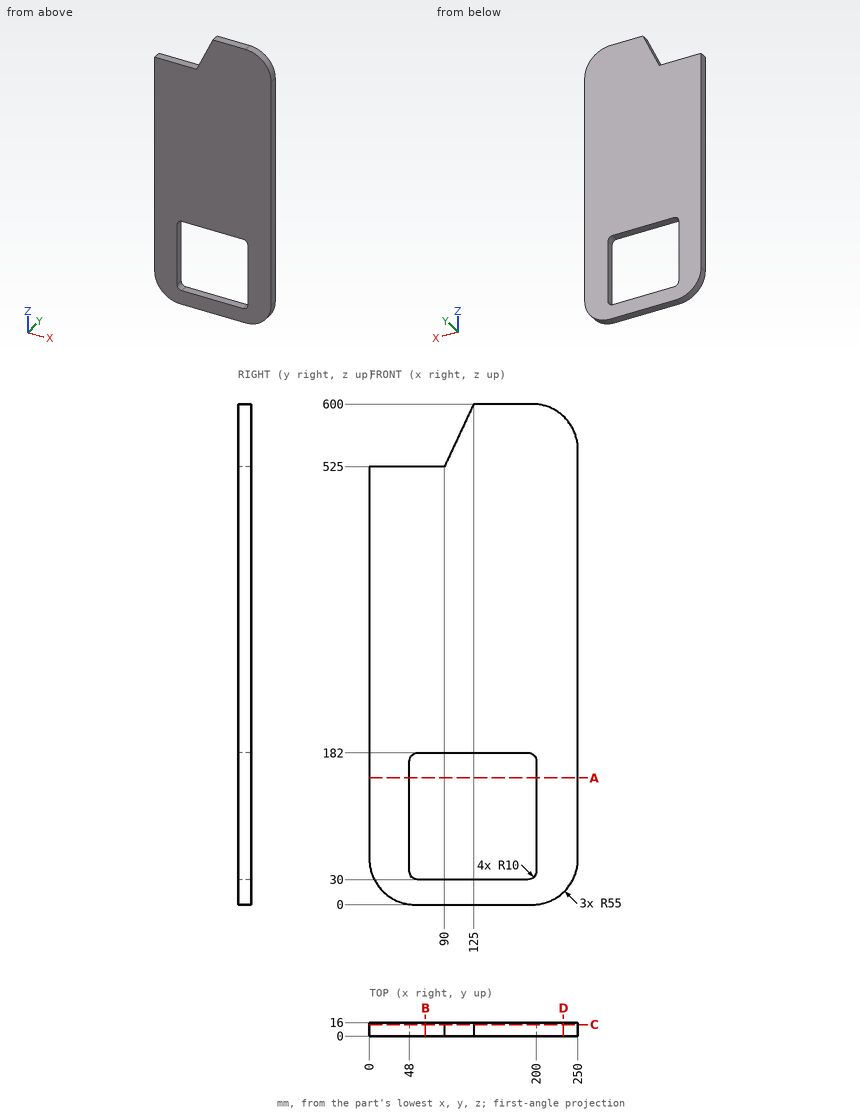
The figure shows three views and two pictorial views of one solid part (mm, origin at its lowest corner). Answer the questions. Round coordinates to 2 decimals unless told otherwise and drop trailing zeros. Write each loop counter-clockwise with the first axis right and the second up, starting at its lowest first coordinate (ties: lowest second). Pieces come first, ordered by that corner, then holes. Notation, with made-up numbers: (24.5, -14) - (58.5, -14) arc R20 ccw to (58.5, 9) - close; hole circle Ø1 at (36, 16.25). An arc over 180 degrees is marked (long way). Answer in a Markdown table with one row per item. Add a question column.
1. A cutting plane is placed at C-C, the plane y = 13.5. Determine the outline of the cut face in (x, z).
2. A cutting plane is placed at D-D, the plane x = 232.5. Determine the outline of the cut face in (y, z).
3. Find the intervals of material crossed by line 1 along Z through (x, y) = (135, 13); line 2 along X through (y, z) = (7, 59); line 3 along Z through (x, y) = (80, 10.5), in increasing order. Write a range as from..to.
4. A cutting plane is placed at B-B, the plane x = 67. Determine the outline of the cut face in (y, z), and give its area (3 significant figures).
5. A cutting plane is placed at A-A, the plane z = 152. Determine the outline of the cut face in (x, y), and give its area (3 significant figures).
6. Given pin 1 (4 mm diameter, centred on x = 31.5, z = 119, fed in from -Y); pin 2 (2 mm diameter, centred on x = 41, y = 7.5, fed in from -Z); pin 3 (5 mm diameter, centred on x = 55, y = 7.5, fed in from +Z), each flat-ended and moving along its own axis, determine where each tip first touches the part or whether it passes through.
Worked out:
| question | item | result |
|---|---|---|
| 1 | outline | (0, 55) arc R55 ccw to (55, 0) - (195, 0) arc R55 ccw to (250, 55) - (250, 545) arc R55 ccw to (195, 600) - (125, 600) - (90, 525) - (0, 525) - close; hole (48, 40) arc R10 ccw to (58, 30) - (190, 30) arc R10 ccw to (200, 40) - (200, 172) arc R10 ccw to (190, 182) - (58, 182) arc R10 ccw to (48, 172) - close |
| 2 | outline | (0, 14.77) - (16, 14.77) - (16, 585.23) - (0, 585.23) - close |
| 3 | line 1 | 0..30, 182..600 |
| 3 | line 2 | 0..48, 200..250 |
| 3 | line 3 | 0..30, 182..525 |
| 4 | outline | (0, 0) - (16, 0) - (16, 30) - (0, 30) - close; (0, 182) - (16, 182) - (16, 525) - (0, 525) - close |
| 4 | area | 5,970 mm^2 |
| 5 | outline | (0, 0) - (48, 0) - (48, 16) - (0, 16) - close; (200, 0) - (250, 0) - (250, 16) - (200, 16) - close |
| 5 | area | 1,570 mm^2 |
| 6 | pin 1 | y = 0 |
| 6 | pin 2 | z = 1.56 |
| 6 | pin 3 | z = 525 |
